Work out the finished part from the listing and answer in its coordinate system (mm). A direction names the side the tool comes from. Round coordinates to 2 decimals unless told otherwise and drop trailing zeros. Write each loop counter-clockwise with the first axis right and the second up, starting at its lowest first coordinate (ties: lowest second). Pieces come first, ordered by that corner, then holes.
1. Find section D-D (z = 17). Write down the section's boundary in (x, y), and give its area (3 significant figures).
2. Straight lines are drawn through the part: probe 1 along Z at (x, y) = (-72, -43.5); probe 2 along X at (y, z) = (-290, 1.05); probe 3 along X at (y, z) = (-211, 18). For each, find the intervals that lie inside material, in ascending order.
3. Find section B-B (x = -45). Write down the section's boundary in (y, z), and give its area (3 significant figures).
4. Find section C-C (y = -114). Write down the section's boundary in (x, z).
5. Determine the mould class of faces 1 (the face through (-45.493, -2.852, 1.233)), 2 (the face through (-59, -148, 32.5)), 3 (the face through (-52.298, -294.216, 31.232)) for opening direction X: pulls with the +X half, pulls with the -X half, needs draft (parallel to the pull), parting line crosses it, or undercut.
6. A tool of negligible diameter and unlimited length cuts with its end or side. For faces 4 (the face through (-45.337, -3.007, 31.232)), 5 (the face through (-72.486, -148, 16)), from which of +Z, -Z, +X, -X, +Y, -Y can it reach the whole face along a straight path? Write none if from no direction.
7. Flat-ended cylindrical pins translate along their axes: pin 1 Ø8 at (x, y) = (-54.99, -10) entering from +Z; pin 2 Ø1 at (y, z) = (-231, 17.5) entering from +X. Find the tip coordinate at first contact, or state that the pin passes through.
8. Find section A-A (y = -260). Write down the section's boundary in (x, z).
```python
from build123d import *

# Parameters (mm, degrees)
F2_DEPTH    = 300
F1_R        = 5
F3_DEPTH    = 46
F4_T1_DEPTH = 52.5
F4_T3_DEPTH = 52.5
F4_T5_DEPTH = 82.5


# Not quite as in the source:
# - a fillet or chamfer that OpenCascade refuses, or shapes differently, is made with other operations: its cross-section is extruded or revolved along the edge and cut away or added
# - a pattern or mirror of a feature is missing from the dataset's text; its kind, count and spacing are read off the source's solid


with BuildPart() as f2:
    # F0 (on Front) → F2 (new body)
    with BuildSketch(Plane.XZ):
        Polygon((-74.9858543277, 32.5), (-74.9858543277, 0), (-42.4858543277, 0), (-42.4858543277, 2.5), (-72.4858543277, 2.5), (-72.4858543277, 30), (-42.4858543277, 30), (-42.4858543277, 32.5), align=None)
    extrude(amount=F2_DEPTH)

    # F1 (on Top) → F3 (cut)
    with BuildSketch(Plane.XY):
        with Locations((-54.9858543277, -260)):
            Circle(F1_R)
        with Locations((-54.9858543277, -40)):
            Circle(F1_R)
        with Locations((-54.9858543277, -10)):
            Circle(F1_R)
    f3 = extrude(amount=F3_DEPTH, mode=Mode.SUBTRACT)

    # F3_copies: F3 across plane
    add(f3.mirror(Plane(origin=(0, -275, 0), x_dir=(0, 0, -1), z_dir=(0, -1, 0))), mode=Mode.SUBTRACT)

    # F4: fillet of radius 10 on 6 edges, made by hand

    # F4_s2 → F4_t1 (cut)
    with BuildSketch(Plane.XY.offset(-25)):
        with BuildLine():
            ThreePointArc((-52.4858543277, 0), (-45.4147865158, -2.9289321881), (-42.4858543277, -10))
            Line((-42.4858543277, -10), (-42.4858543277, 0))
            Line((-42.4858543277, 0), (-52.4858543277, 0))
        make_face()
        with BuildLine():
            ThreePointArc((-52.4858543277, -300), (-45.4147865158, -297.0710678119), (-42.4858543277, -290))
            Line((-42.4858543277, -290), (-42.4858543277, -300))
            Line((-42.4858543277, -300), (-52.4858543277, -300))
        make_face()
    extrude(amount=F4_T1_DEPTH, mode=Mode.SUBTRACT)

    # F4_s4 → F4_t3 (cut)
    with BuildSketch(Plane.XY.offset(5)):
        with BuildLine():
            ThreePointArc((-42.4858543277, -10), (-45.4147865158, -2.9289321881), (-52.4858543277, 0))
            Line((-52.4858543277, 0), (-42.4858543277, 0))
            Line((-42.4858543277, 0), (-42.4858543277, -10))
        make_face()
        with BuildLine():
            ThreePointArc((-42.4858543277, -290), (-45.4147865158, -297.0710678119), (-52.4858543277, -300))
            Line((-52.4858543277, -300), (-42.4858543277, -300))
            Line((-42.4858543277, -300), (-42.4858543277, -290))
        make_face()
    extrude(amount=F4_T3_DEPTH, mode=Mode.SUBTRACT)

    # F4_s6 → F4_t5 (cut)
    with BuildSketch(Plane.XY.offset(-25)):
        with BuildLine():
            ThreePointArc((-64.9858543277, 0), (-72.0569221395, -2.9289321881), (-74.9858543277, -10))
            Line((-74.9858543277, -10), (-74.9858543277, 0))
            Line((-74.9858543277, 0), (-64.9858543277, 0))
        make_face()
        with BuildLine():
            ThreePointArc((-64.9858543277, -300), (-72.0569221395, -297.0710678119), (-74.9858543277, -290))
            Line((-74.9858543277, -290), (-74.9858543277, -300))
            Line((-74.9858543277, -300), (-64.9858543277, -300))
        make_face()
    extrude(amount=F4_T5_DEPTH, mode=Mode.SUBTRACT)


solid = f2.part
```
Worked answers:
1. outline: (-74.99, -290) arc R10 ccw to (-72.49, -296.61) - (-72.49, -3.39) arc R10 ccw to (-74.99, -10) - close
1. area: 723 mm2
2. probe 1: z = 0 to 2.5, 30 to 32.5
2. probe 2: x = -74.99 to -59.99, -49.99 to -42.49
2. probe 3: x = -74.99 to -72.49
3. outline: (-296.63, 0) - (-3.37, 0) - (-3.37, 2.5) - (-296.63, 2.5) - close; (-296.63, 30) - (-3.37, 30) - (-3.37, 32.5) - (-296.63, 32.5) - close
3. area: 1,470 mm2
4. outline: (-74.99, 0) - (-42.49, 0) - (-42.49, 2.5) - (-72.49, 2.5) - (-72.49, 30) - (-42.49, 30) - (-42.49, 32.5) - (-74.99, 32.5) - close
5. face 1: pulls with the +X half
5. face 2: needs draft
5. face 3: undercut
6. face 4: +Z, -Z, +X, +Y
6. face 5: +X, +Y, -Y
7. pin 1: passes through
7. pin 2: stops at x = -72.49
8. outline: (-74.99, 0) - (-59.99, 0) - (-59.99, 2.5) - (-72.49, 2.5) - (-72.49, 30) - (-59.99, 30) - (-59.99, 32.5) - (-74.99, 32.5) - close; (-49.99, 0) - (-42.49, 0) - (-42.49, 2.5) - (-49.99, 2.5) - close; (-49.99, 30) - (-42.49, 30) - (-42.49, 32.5) - (-49.99, 32.5) - close
